Geometry: see drawing. Coordinates: mm, zero at the bounding-box minimum. A direction names the side the tool comes from. Round coordinates to 2 decimals unless told otherwise and drop trailing zeros. Order: outer loops, then holes, each group sorted by start corner. A loop starts at its lowest first (then second) coordinate and runs counter-clockwise, first axis right, second up. Notation, with made-up numbers: (-10.5, 71.5) - (11.5, 71.5) arc R28 ccw to (11.5, 98.5) - close; hole circle Ø4 at (-1, 17). An arc over 180 degrees is marked (long way). Put each result on its own line as item: value. Start each with the question number.
1) Line query: probe 1 along Z at (x, y) = (25, 11.75); probe 2 along X at (y, z) = (3, 24); probe 3 along Z at (x, y) = (10.75, 12.5). Output: solid intervals per line, ascending. Write a range as [from, to].
2) Section D-D on z = 25.5. Output: boundary loops of the cut face in (x, y), then the cut area to 3 significant figures.
3) Section B-B on y = 7.5. State how many separate pieces and enclosed holes the cut face has, then the cut area to 3 significant figures.
4) Section A-A on x = 10.75. Output: boundary loops of the cut face in (y, z).
5) Access query for the marked faces 1, 2, 3, 4 and 5. Directions: +Z, -Z, +X, -X, +Y, -Y. A direction counts if a zero-diameter tool reaches every point of the face in a straight line with its end or side. Return the directions, or none.
6) Section C-C on x = 22. Output: boundary loops of the cut face in (y, z).
7) Mould query, pull axis X, two halves, no side actions, for the marked faces 6, 7, 8 and 9. Classes: +X half, -X half, draft (parallel to the pull), parting line (faces both ways), or undercut.
8) Contact query for flat-ended pins moving along their axis: P1, Ø1.5, axis at y = 6, z = 3.5, coming from the +X side; P2, Ø7.5, axis at x = 19.5, y = 10, coming from the +Z side; P3, Ø1.4, axis at y = 8, z = 25.5, coming from the +X side. Output: stop coordinate, or through.
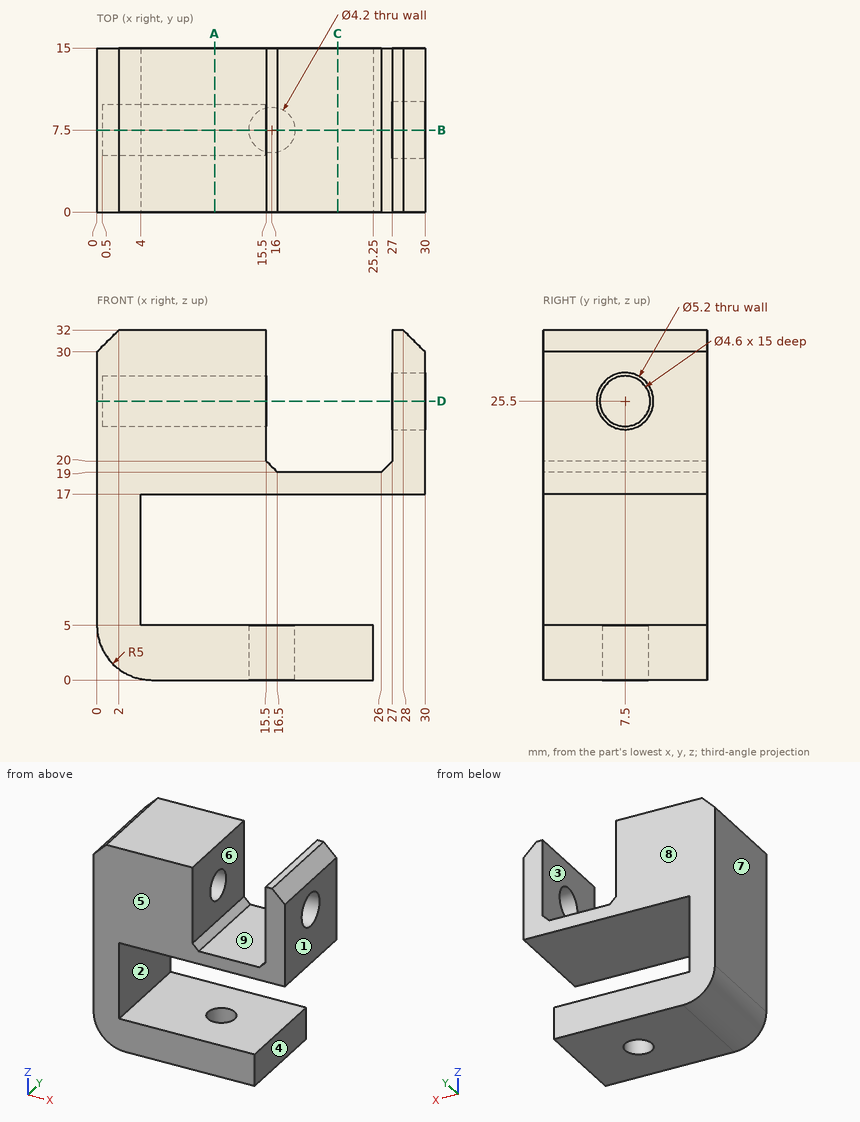
Answer sheet:
1. probe 1: [0, 5], [17, 19]
1. probe 2: [0, 15.5], [27, 30]
1. probe 3: [0, 5], [17, 32]
2. outline: (0, 0) - (15.5, 0) - (15.5, 5.2) - (0.5, 5.2) - (0.5, 9.8) - (15.5, 9.8) - (15.5, 15) - (0, 15) - close; (27, 0) - (30, 0) - (30, 4.9) - (27, 4.9) - close; (27, 10.1) - (30, 10.1) - (30, 15) - (27, 15) - close
2. area: 193 mm^2
3. separate pieces: 3
3. enclosed holes: 0
3. area: 361 mm^2
4. outline: (0, 0) - (15, 0) - (15, 5) - (0, 5) - close; (0, 17) - (15, 17) - (15, 32) - (0, 32) - close; hole circle Ø4.6 at (7.5, 25.5)
5. face 1: +Z, -Z, +X, +Y, -Y
5. face 2: +X, +Y, -Y
5. face 3: +Z, +Y, -Y
5. face 4: -Z, +X, +Y, -Y
5. face 5: +Z, -Z, +X, -X, -Y
6. outline: (0, 0) - (15, 0) - (15, 5) - (0, 5) - close; (0, 17) - (15, 17) - (15, 19) - (0, 19) - close
7. face 6: undercut
7. face 7: -X half
7. face 8: draft
7. face 9: undercut
8. P1: x = 25.25
8. P2: z = 19.75
8. P3: x = 0.5
